Could you check a few things on this model? Use its own coordinates, in mm. Face numbers are marked on the shaded views. A direction names the side the tool comes from. Give positions to 0.01 mm unless a question says otherwise; leave off trailing zeros. Order: outer loops, then holes, each group sorted by start corner. A loop starts at its lowest first (then second) coordinate and runs counter-clockwise, first axis right, second up. Notation, with made-up numbers: (9.5, 56) -> (56.5, 56) arc R7 cw to (56.5, 66) -> close; hole circle Ø8 at (69.25, 30). An arc over 180 degrees is marked (long way). Use one line per item in the form item = value. Start each with the question number.
from build123d import *

# Parameters (mm, degrees)
SKETCH1_R           = 2
BOSS_EXTRUDE1_DEPTH = 2
SKETCH2_R           = 4
BOSS_EXTRUDE2_DEPTH = 2
BOSS_EXTRUDE3_DEPTH = 2
SKETCH4_R           = 6
BOSS_EXTRUDE4_DEPTH = 2


with BuildPart() as part:
    # Sketch1 → Boss-Extrude1 (new body)
    with BuildSketch(Plane.XY):
        Circle(SKETCH1_R)
    extrude(amount=BOSS_EXTRUDE1_DEPTH)

    # Sketch2 → Boss-Extrude2 (add)
    with BuildSketch(Plane(origin=(0, 0, 0), x_dir=(-1, 0, 0), z_dir=(0, 0, -1))):
        Circle(SKETCH2_R)
    extrude(amount=BOSS_EXTRUDE2_DEPTH)

    # Sketch3 → Boss-Extrude3 (add)
    with BuildSketch(Plane(origin=(0, 0, -2), x_dir=(-1, 0, 0), z_dir=(0, 0, -1))):
        Polygon((21.988055025, 12.156292042), (-0.985889756, 2.297394478), (0.985889756, -2.297394478), (23.959834538, 7.561503086), align=None)
    extrude(amount=BOSS_EXTRUDE3_DEPTH)

    # Sketch4 → Boss-Extrude4 (add)
    with BuildSketch(Plane.XY.offset(-2)):
        with Locations(Location((-22.973944782, 9.858897564, 0), (0, 0, 312.149872239))):
            Circle(SKETCH4_R)
    extrude(amount=BOSS_EXTRUDE4_DEPTH)


solid = part.part
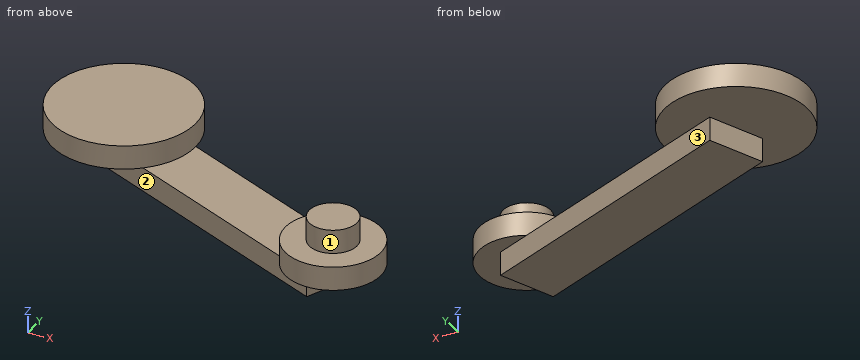
(1) Imagine slicing it at B-B (z = 1.1). Write out the boundary of the cut face in (x, y), plus the area to 3 significant figures.
(2) Imagine slicing it at C-C (y = 0). Write out the boundary of the cut face in (x, z).
(3) Imagine slicing it at D-D (x = -1.5). Write out the boundary of the cut face in (y, z).
(4) Imagine slicing it at A-A (y = 5). Write out the boundary of the cut face in (x, z), plus the area to 3 significant figures.
(5) Please list where these lines run through material, in increasing order: probe 1 along Y at (x, z) = (0, -1.5); probe 2 along Z at (x, y) = (-22, 14.25); probe 3 along Z at (x, y) = (-0.5, -1.5).
(6) I'm going to push flat-ended pins straight in: pin 1 Ø2 at (x, y) = (-2, 4) entering from +Z; pin 2 Ø3.5 at (x, y) = (-10, 3) entering from +Z; pin 3 Ø1 at (y, z) = (1, -2) entering from -X. Where does each tip first touch, or does it pass through?
(7) Which directions (+Z, -Z, +X, -X, +Y, -Y) give clear straight access to the entire face, cutting with the end or side of a thin tool? Please do the marked faces 1, 2 and 3.
Calculated:
q1.outline = circle Ø4 at (0, 0)
q1.area = 12.6 mm2
q2.outline = (-6.34, -4) -> (0, -4) -> (0, -2) -> (4, -2) -> (4, 0) -> (2, 0) -> (2, 2) -> (-2, 2) -> (-2, 0) -> (-4, 0) -> (-4, -2) -> (-6.34, -2) -> close
q3.outline = (-3.71, -2) -> (-2.08, -2) -> (-2.08, -4) -> (3.36, -4) -> (3.36, -2) -> (3.71, -2) -> (3.71, 0) -> (1.32, 0) -> (1.32, 2) -> (-1.32, 2) -> (-1.32, 0) -> (-3.71, 0) -> close
q4.outline = (-26.49, -2) -> (-19.45, -2) -> (-19.45, 0) -> (-26.49, 0) -> close; (-17.99, -4) -> (-5.31, -4) -> (-5.31, -2) -> (-17.99, -2) -> close
q4.area = 39.4 mm2
q5.probe_1 = -4 to 4
q5.probe_2 = -2 to 0
q5.probe_3 = -2 to 2
q6.pin_1 = 0
q6.pin_2 = -2
q6.pin_3 = -9.83
q7.face_1 = +Z
q7.face_2 = -Z, -X, -Y
q7.face_3 = -Z, +X, +Y
